Check sheet for the modelled part. Datum: model origin and axes. Units: mm. Round coordinates to 2 decimals unless told otherwise and drop trailing zeros. Loops run counter-clockwise (first coordinate to the right, second up) from the corner with the lowest first, then second, coordinate; pieces in that order, holes last. Notation, with made-up numbers: (74, 37) -> (117, 37) arc R20 cw to (117, 66) -> close; hole circle Ø3 at (22, 54). An arc over 180 degrees is marked (long way). One line per item, written item: value. Start each with the question number.
1. Material ranges on L1, parallel to Z at x = 0, y = 1.25; L2, parallel to Z at x = -1, y = 1.75; L3, parallel to Z at x = 1.25, y = 1.45, recorded low to high.
2. Cross-section at A-A on y = 1.5. Record the cut outline in (x, z), then the cut area to 3 significant figures.
3. Cross-section at B-B on z = -1. Record the cut outline in (x, y).
4. Cross-section at C-C on z = 9. Record the cut outline in (x, y), then the cut area to 3 significant figures.
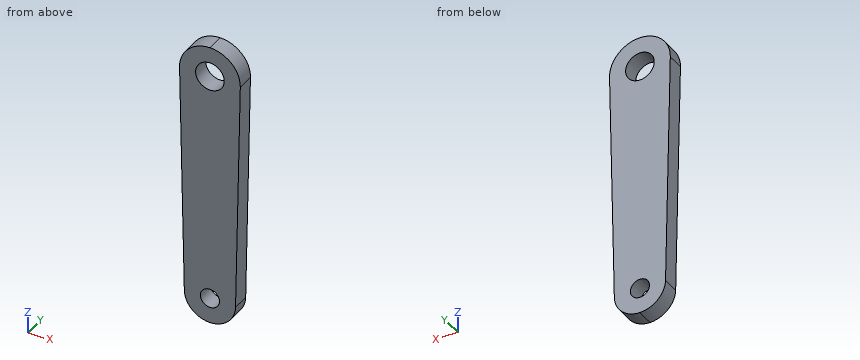
Autodesk Inventor part; units mm, degrees
ref_plane "YZ Plane" through (0, 0, 0) normal (1, 0, 0) x (0, 1, 0)
ref_plane "XZ Plane" through (0, 0, 0) normal (0, 1, 0) x (-1, 0, 0)
ref_plane "XY Plane" through (0, 0, 0) normal (0, 0, 1) x (1, 0, 0)
sketch "Эскиз1" plane through (0, 0, 0) normal (0, 1, 0) x (-1, 0, 0)
  line L0 (0, 17) -> (0, 17)
  line L1 (0, -17) -> (0, -17)
  arc A0 (3.4993, 13.4287) -> (0, 17) centre (0, 13.5) ccw
  circle A1 centre (0, 13.5) radius 1.65
  circle A2 centre (0, -13.5) radius 1.1
  line L2 (3.4993, 13.4287) -> (2.9494, -13.5601)
  arc A3 (0, -16.45) -> (2.9494, -13.5601) centre (0, -13.5) ccw
  arc A4 (0, 17) -> (-3.4993, 13.4287) centre (0, 13.5) ccw
  line L3 (-3.4993, 13.4287) -> (-2.9494, -13.5601)
  arc A5 (-2.9494, -13.5601) -> (0, -16.45) centre (0, -13.5) ccw
  point P0 (0, 0)
  dimension "d2" = 3.5
  dimension "d4" = 2.2
  dimension "d5" = 3.3
extrude "Выдавливание1" add sketch "Эскиз1" along normal blind 2
properties part number "servo_leg"
Taken from the geometry:
1. L1: z = -16.45 to -14.6, -12.4 to 11.85, 15.15 to 17
1. L2: z = -16.28 to -13.96, -13.04 to 12.19, 14.81 to 16.85
1. L3: z = -16.17 to 12.42, 14.58 to 16.77
2. outline: (-3.5, 13.43) -> (-2.95, -13.56) arc R2.95 ccw to (0, -16.45) arc R2.95 ccw to (2.95, -13.56) -> (3.5, 13.43) arc R3.5 ccw to (0, 17) arc R3.5 ccw to start; hole circle Ø3.3 at (0, 13.5); hole circle Ø2.2 at (0, -13.5)
2. area: 195 mm2
3. outline: (-3.21, 0) -> (3.21, 0) -> (3.21, 2) -> (-3.21, 2) -> close
4. outline: (-3.41, 0) -> (3.41, 0) -> (3.41, 2) -> (-3.41, 2) -> close
4. area: 13.6 mm2
